from build123d import *

# Parameters (mm, degrees)
F1_DEPTH       = 8
F3_D           = 4
F3_CSINK_D     = 5
F3_CSINK_ANGLE = 90
F4_R           = 1


with BuildPart() as f1:
    # F0 (on Front) → F1 (new body, symmetric)
    with BuildSketch(Plane.XZ):
        with BuildLine():
            Line((0, -5.3220339234), (24.75, -5.3220339234))
            Line((24.75, -5.3220339234), (24.75, 2.6779660766))
            Line((24.75, 2.6779660766), (12.75, 2.6779660766))
            Line((12.75, 2.6779660766), (12.75, 38.6779660766))
            Line((12.75, 38.6779660766), (1.5, 38.6779660766))
            Line((1.5, 38.6779660766), (1.5, 31.5360828994))
            ThreePointArc((1.5, 31.5360828994), (7.964450219, 22.9246184085), (0, 15.6779660766))
            Line((0, 15.6779660766), (0, -5.3220339234))
        make_face()
        with BuildLine():
            Line((-24.75, -5.3220339234), (0, -5.3220339234))
            Line((0, -5.3220339234), (0, 15.6779660766))
            ThreePointArc((0, 15.6779660766), (-7.964450219, 22.9246184085), (-1.5, 31.5360828994))
            Line((-1.5, 31.5360828994), (-1.5, 38.6779660766))
            Line((-1.5, 38.6779660766), (-12.75, 38.6779660766))
            Line((-12.75, 38.6779660766), (-12.75, 2.6779660766))
            Line((-12.75, 2.6779660766), (-24.75, 2.6779660766))
            Line((-24.75, 2.6779660766), (-24.75, -5.3220339234))
        make_face()
    extrude(amount=F1_DEPTH, both=True)

    # F3 (through all)
    with Locations(Plane.XY.offset(2.6779660766)):
        with Locations((18.75, 0), (-18.75, 0)):
            CounterSinkHole(F3_D / 2, F3_CSINK_D / 2, counter_sink_angle=F3_CSINK_ANGLE)

    # F4
    f4_edges = [f1.edges().sort_by_distance(p)[0] for p in [
        (-12.75, -8, 20.677966),
        (-7.125, -8, 38.677966),
        (7.125, -8, 38.677966),
        (12.75, -8, 20.677966),
        (18.75, -8, 2.677966),
        (-18.75, -8, 2.677966),
        (24.75, -8, -1.322034),
        (-24.75, -8, -1.322034),
        (12.75, 0, 2.677966),
        (24.75, 0, 2.677966),
        (24.75, 8, -1.322034),
        (12.75, 8, 20.677966),
        (1.5, 8, 35.107024),
        (-1.5, 8, 35.107024),
        (1.5, 0, 31.536083),
        (0, 8, 15.677966),
        (-1.5, 0, 31.536083),
        (0, -8, 15.677966),
        (-7.125, 8, 38.677966),
        (-12.75, 8, 20.677966),
        (-18.75, 8, 2.677966),
        (-24.75, 8, -1.322034),
        (-24.75, 0, 2.677966),
        (18.75, 8, 2.677966),
    ]]
    fillet(f4_edges, radius=F4_R)


solid = f1.part
Read the model definition and answer for the solid it produces. Units are mm, in the model's axes. A direction names the side the tool comes from. Give positions to 0.01 mm unless a question says otherwise; leave off trailing zeros. Loops run counter-clockwise (first coordinate to the right, second up) from the corner with the lowest first, then second, coordinate; pieces in that order, holes last. Notation, with made-up numbers: (72.25, 49.25) -> (86.25, 49.25) arc R9 ccw to (86.25, 62.25) -> close; hole circle Ø3 at (-24, -36). An arc over 180 degrees is marked (long way). Use a Markdown table: item, result.
Q1. Determine the mould class of faces 1 (the face through (12.75, 0, 21)), 2 (the face through (0, -8, 12)), 3 (the face through (20.337, -1.217, -1.625)) for opening direction X: pulls with the +X half, pulls with the -X half, needs draft (parallel to the pull), parting line crosses it, or undercut.
Solved:
| item | result |
|---|---|
| face 1 | pulls with the +X half |
| face 2 | needs draft |
| face 3 | undercut |
Q2. Find the intervals of material crossed by line 1 along X through (y, z) = (0, -1.5); line 2 along Y through (x, z) = (18.75, -1); line 3 along X through (y, z) = (2.25, 35), in increasing order.
Solved:
| item | result |
|---|---|
| line 1 | x = -24.75 to -20.75, -16.75 to 16.75, 20.75 to 24.75 |
| line 2 | y = -8 to -2, 2 to 8 |
| line 3 | x = -12.75 to -1.5, 1.5 to 12.75 |
Q3. A tool of negligible diameter and unlimited length cuts with its end or side. For faces 4 (the face through (-12.75, 0, 21)), 5 (the face through (-1.5, -1, 35)), 6 (the face through (0, 8, 12)), 7 (the face through (21, -2, 2.678)), from which of +Z, -Z, +X, -X, +Y, -Y can it reach the whole face along a straight path? Write none if from no direction.
Solved:
| item | result |
|---|---|
| face 4 | +Z, -X, +Y, -Y |
| face 5 | +Z, +Y, -Y |
| face 6 | +Z, -Z, +X, -X, +Y |
| face 7 | +Z, +X, +Y, -Y |
Q4. Section D-D, the plane y = 5.25 is taken. Determine the outline of the cut face in (x, z).
Solved:
| item | result |
|---|---|
| outline | (-24.75, -5.32) -> (24.75, -5.32) -> (24.75, 1.68) arc R1 ccw to (23.75, 2.68) -> (13.75, 2.68) arc R1 cw to (12.75, 3.68) -> (12.75, 38.68) -> (1.5, 38.68) -> (1.5, 32.32) arc R1 ccw to (2.22, 31.36) arc R8 cw (long way) to (-2.22, 31.36) arc R1 ccw to (-1.5, 32.32) -> (-1.5, 38.68) -> (-12.75, 38.68) -> (-12.75, 2.68) -> (-23.75, 2.68) arc R1 ccw to (-24.75, 1.68) -> close |
Q5. Section B-B, the plane x = 18.75 is taken. Determine the outline of the cut face in (y, z), then the cut area to 3 significant figures.
Solved:
| item | result |
|---|---|
| outline | (-8, -5.32) -> (-2, -5.32) -> (-2, 2.18) -> (-2.5, 2.68) -> (-7, 2.68) arc R1 ccw to (-8, 1.68) -> close; (2, -5.32) -> (8, -5.32) -> (8, 1.68) arc R1 ccw to (7, 2.68) -> (2.5, 2.68) -> (2, 2.18) -> close |
| area | 95.3 mm^2 |
Q6. Section C-C, the plane y = 0 is taken. Count the separate pieces of the cut face and the enclosed holes in it, then the cut area to 3 significant figures.
Solved:
| item | result |
|---|---|
| separate pieces | 3 |
| enclosed holes | 0 |
| area | 1,030 mm^2 |
Q7. Section A-A, the plane z = 33.5 is taken. Determine the outline of the cut face in (x, y).
Solved:
| item | result |
|---|---|
| outline | (-12.75, -7) arc R1 ccw to (-11.75, -8) -> (-1.5, -8) -> (-1.5, 7) arc R1 ccw to (-2.5, 8) -> (-11.75, 8) arc R1 ccw to (-12.75, 7) -> close; (1.5, -8) -> (11.75, -8) arc R1 ccw to (12.75, -7) -> (12.75, 7) arc R1 ccw to (11.75, 8) -> (2.5, 8) arc R1 ccw to (1.5, 7) -> close |
Q8. Each of these flat-tipped pins is pushed along its axis until it touches: pin 1 (5.5 mm diameter, centred on x = -19, y = 2, fed in from +Z); pin 2 (7 mm diameter, centred on y = 0, z = 36.5, fed in from -X); pin 3 (6 mm diameter, centred on y = -4.5, z = 28, fed in from +X); pin 4 (3.5 mm diameter, centred on x = 18.75, y = 0, fed in from -Z). Where does it stop, or does it pass through?
Solved:
| item | result |
|---|---|
| pin 1 | stops at z = 2.68 |
| pin 2 | stops at x = -12.75 |
| pin 3 | stops at x = 12.75 |
| pin 4 | passes through |
